Geometry check sheet. Reference: the model listing, model coordinates, mm. Face numbers are marked on the shaded views. A direction names the side the tool comes from. Coordinates: 2 decimals unless noted, no trailing zeros. Write each loop counter-clockwise with the first axis right and the second up, starting at its lowest first coordinate (ties: lowest second). Pieces come first, ordered by that corner, then holes. Notation, with made-up numbers: (-26, -11.5) -> (0, -11.5) arc R18 cw to (0, -0.5) -> close; hole circle Ø3 at (10, 43.25). An arc over 180 degrees is marked (long way). One line per question, with ' | ' between items.
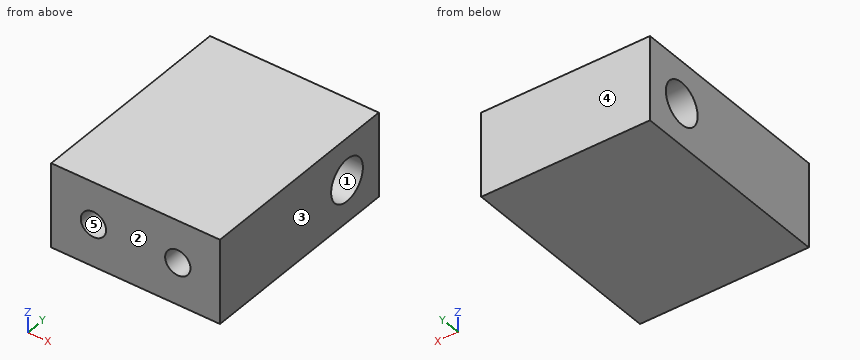
```python
from build123d import *

# Parameters (mm, degrees)
SKETCH1_W           = 20
SKETCH1_H           = 10
BOSS_EXTRUDE1_DEPTH = 25
SKETCH2_R           = 1.5
CUT_EXTRUDE1_DEPTH  = 10
SKETCH3_R           = 2.5
CUT_EXTRUDE2_DEPTH  = 20


with BuildPart() as part:
    # Sketch1 → Boss-Extrude1 (new body)
    with BuildSketch(Plane(origin=(0, 0, 0), x_dir=(1, 0, 0), z_dir=(0, 1, 0))):
        Rectangle(SKETCH1_W, SKETCH1_H)
    extrude(amount=BOSS_EXTRUDE1_DEPTH)

    # Sketch2 → Cut-Extrude1 (cut)
    with BuildSketch(Plane(origin=(0, 0, 0), x_dir=(1, 0, 0), z_dir=(0, 1, 0))):
        with Locations(Location((-5, 0, 0), (0, 0, 270))):
            Circle(SKETCH2_R)
        with Locations(Location((5, 0, 0), (0, 0, 270))):
            Circle(SKETCH2_R)
    extrude(amount=CUT_EXTRUDE1_DEPTH, mode=Mode.SUBTRACT)

    # Sketch3 → Cut-Extrude2 (cut, symmetric)
    with BuildSketch(Plane(origin=(0, 0, 0), x_dir=(0, 0, -1), z_dir=(1, 0, 0))):
        with Locations((0, 20)):
            Circle(SKETCH3_R)
    extrude(amount=CUT_EXTRUDE2_DEPTH, both=True, mode=Mode.SUBTRACT)


solid = part.part
```
(1) Cross-section at D-D (y = 2.75). Record the cut outline in (x, z).
Answers below:
outline: (-10, -5) -> (10, -5) -> (10, 5) -> (-10, 5) -> close; hole circle Ø3 at (-5, 0); hole circle Ø3 at (5, 0)
(2) Cross-section at C-C (x = -5). Record the cut outline in (y, z).
Answers below:
outline: (0, -5) -> (25, -5) -> (25, 5) -> (0, 5) -> (0, 1.5) -> (10, 1.5) -> (10, -1.5) -> (0, -1.5) -> close; hole circle Ø5 at (20, 0)
(3) Cross-section at B-B (z = 0). Record the cut outline in (x, y), plus the area to 3 significant figures.
Answers below:
outline: (-10, 0) -> (-6.5, 0) -> (-6.5, 10) -> (-3.5, 10) -> (-3.5, 0) -> (3.5, 0) -> (3.5, 10) -> (6.5, 10) -> (6.5, 0) -> (10, 0) -> (10, 17.5) -> (-10, 17.5) -> close; (-10, 22.5) -> (10, 22.5) -> (10, 25) -> (-10, 25) -> close | area: 340 mm²
(4) Material ranges on line 1 (X direction, y = 6.25, z = 0); line 2 (X direction, y = 8.25, z = -0.5); line 3 (Y direction, x = 8.75, z = -0.5), recorded low to high.
Answers below:
line 1: x = -10 to -6.5, -3.5 to 3.5, 6.5 to 10 | line 2: x = -10 to -6.41, -3.59 to 3.59, 6.41 to 10 | line 3: y = 0 to 17.55, 22.45 to 25
(5) Tool access check on the marked faces 4 and 5. Record the directions out of +Z, -Z, +X, -X, +Y, -Y that give a thin tool (end or side, any length) a straight path to the whole face; none if there is none.
Answers below:
face 4: +Z, -Z, +X, -X, +Y | face 5: -Y
(6) Draft check along Y on the marked faces 1, 2 and 3. Enter one of: pulls with the +Y half, pulls with the -Y half, needs draft (parallel to the pull), parting line crosses it, or undercut.
Answers below:
face 1: undercut | face 2: pulls with the -Y half | face 3: needs draft
(7) Depth check by flat-ended pin: P1, Ø1.8, axis at x = -5, z = 0, coming from the -Y side; P2, Ø3, axis at x = 4, z = -2.5, coming from the -Y side. Enter the tip coordinate at first touch or a pass-through.
Answers below:
P1: stops at y = 10 | P2: stops at y = 0
(8) Cross-section at A-A (y = 20). Record the cut outline in (x, z).
Answers below:
outline: (-10, -5) -> (10, -5) -> (10, -2.5) -> (-10, -2.5) -> close; (-10, 2.5) -> (10, 2.5) -> (10, 5) -> (-10, 5) -> close
